Design review of the part shown in the three views and the two pictorial views. Dimensions are in mm from the part's minimum x, y and z. A direction names the side the tool comes from. Coordinates: 2 decimals unless noted, no trailing zeros. Write each loop counter-clockwise with the first axis right and the second up, starting at its lowest first coordinate (ties: lowest second). Pieces come first, ordered by that corner, then holes.
Q1. Take a section at B-B, the plane x = 40.5. Write out the cut boundary in (y, z).
Q2. The part is to be moulded in two halves that separate along Y. For the marked faces 1, 2 and 3, say which applies: released by +Y, released by -Y, zero draft, split by the parting line, or undercut.
Q3. For pin 1 Ø13 at (x, z) = (65, 111.5) entering from -Y, flat-tipped, find the tip position at first contact; note if it passes through.
Q4. For L1, parallel to Y at x = 84, z = 108; L2, parallel to Z at x = 60, y = 351, list the stretches that pass through material, from the lowest coordinate up.
Q5. For the marked faces 4, 5 and 6, list the 3-axis set-ups (+Z, -Z, +X, -X, +Y, -Y) from which the entire face can be reached by the end or side of a thin tool; tool diameter is ignored.
Q6. Take a section at A-A, the plane z = 106.5. Write out the cut boundary in (x, y).
Q7. Take a section at C-C, the plane y = 84.5. Write out the cut boundary in (x, z), plus the area to 3 significant figures.
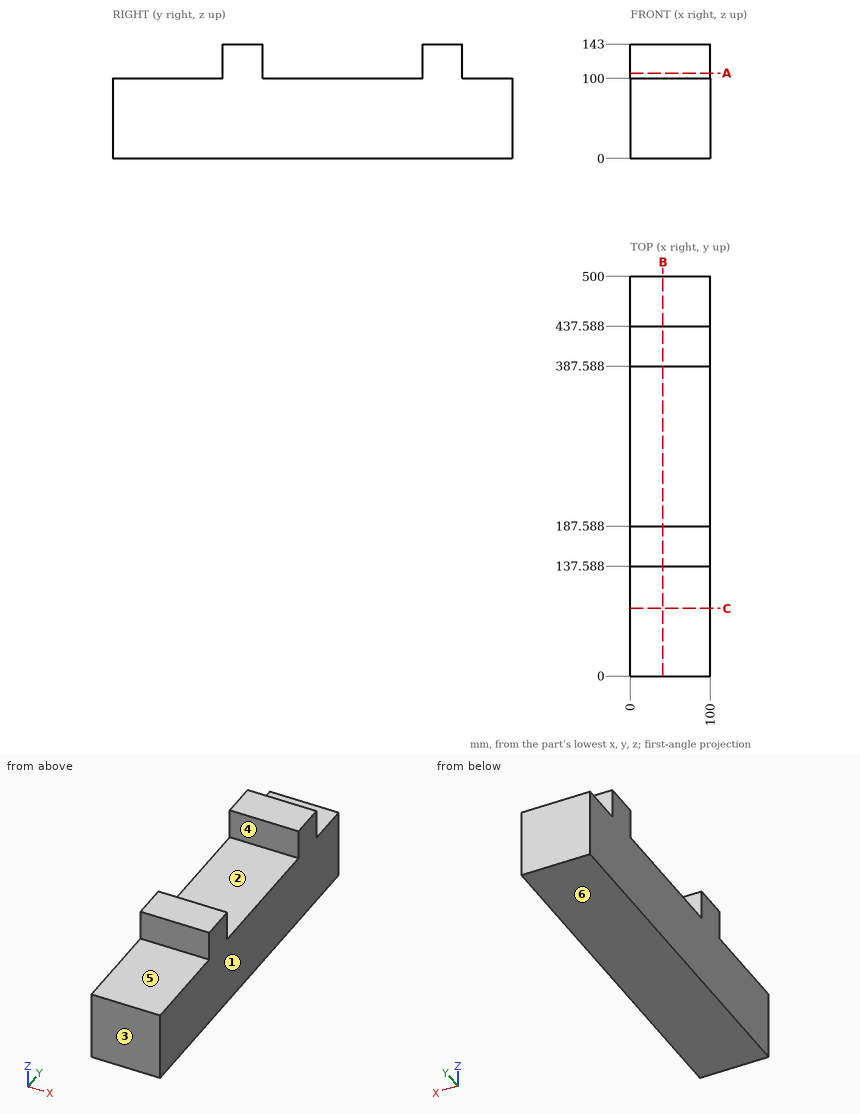
Responses:
1. outline: (0, 0) - (500, 0) - (500, 100) - (437.59, 100) - (437.59, 143) - (387.59, 143) - (387.59, 100) - (187.59, 100) - (187.59, 143) - (137.59, 143) - (137.59, 100) - (0, 100) - close
2. face 1: zero draft
2. face 2: undercut
2. face 3: released by -Y
3. pin 1: stops at y = 137.59
4. L1: y = 137.59 to 187.59, 387.59 to 437.59
4. L2: z = 0 to 100
5. face 4: +Z, +X, -X
5. face 5: +Z, +X, -X, -Y
5. face 6: -Z, +X, -X, +Y, -Y
6. outline: (0, 137.59) - (100, 137.59) - (100, 187.59) - (0, 187.59) - close; (0, 387.59) - (100, 387.59) - (100, 437.59) - (0, 437.59) - close
7. outline: (0, 0) - (100, 0) - (100, 100) - (0, 100) - close
7. area: 10,000 mm2
